Verification items for the finished model (mm, model axes). A direction names the side the tool comes from. Coordinates: 2 decimals unless noted, no trailing zeros. Order: outer loops, then holes, each group sorted by start corner. A loop starts at its lowest first (then second) coordinate and runs counter-clockwise, first axis right, second up. Notation, with made-up numbers: M 32.5,52 L 50.5,52 A30 ccw 50.5,80 Z; hole C 54.25,-25 d6. An arc over 180 degrees is marked long. Return JSON: item names as keys, results as strings. Group by question number.
Q1. Mould release check, pull along Y, two halves, no side actions. Record for faces 1 (the face through (8, -32.329, 4)), 2 (the face through (-36, 37.671, 4)), 3 (the face through (-36.58, 25.84, 2.46)): pulls with the +Y half, pulls with the -Y half, needs draft (parallel to the pull), parting line crosses it, or undercut.
Q2. Section check A-A, the plane x = -2.5. Enter the section's corners in (y, z), then the cut area to 4 significant figures.
Q3. Access from +Z, -Z, +X, -X, +Y, -Y to the whole of each face (thin tool, end or side, straight path). Record for faces 4 (the face through (30.98, 9.22, 4.42)), 5 (the face through (37.73, -28.88, 3.13)), 6 (the face through (14, -12, 2.5)).
Q4. Thickness scan on probe 1 along X at (y, z) = (7.75, 3.75); probe 2 along X at (y, z) = (-15, 4.5); probe 3 along Y at (x, z) = (-27.5, 3). Record the ranges inside material, lowest first.
Q5. Go/stop test with flat-tipped pins: pin 1 Ø4 at (x, z) = (67.61, 3.8) entering from +Y; pin 2 Ø19 at (x, y) = (-35.89, 17.67) entering from -Z; pin 3 Ø3 at (x, z) = (36.11, 3.8) entering from -Y; pin 4 Ø1.8 at (x, y) = (-35.89, 27.17) entering from +Z. Record where each tip stops, or that it passes through.
Q6. Section check B-B, the plane x = 48. Enter the section's corners in (y, z).
from build123d import *

# Parameters (mm, degrees)
BOSS_EXTRU_1_DEPTH       = 7.5
REPOSE_MOTEUR_DEPTH      = 8
ESQUISSE5_R              = 8
FIXATION_COURROI_1_DEPTH = 5
ESQUISSE6_R              = 5.5
FIXATION_COURROI_2_DEPTH = 2.5
ESQUISSE3_R              = 1.5
ESQUISSE3_R_2            = 6
FIXATION_MOTEUR_1_DEPTH  = 5
ESQUISSE2_R              = 13.5
FIXATION_MOTEUR_2_DEPTH  = 2.5
ESQUISSE9_R              = 1.75
PERCAGE_1_DEPTH          = 7
ESQUISSE7_R              = 1.75
PERCAGE_2_DEPTH          = 7


with BuildPart() as part:
    # Esquisse1 → Boss.-Extru.1 (new body)
    with BuildSketch(Plane.XY):
        Polygon((-53.385579659, 37.671052632), (-53.385579659, -32.328947368), (71.614420341, -32.328947368), (71.614420341, 12.671052632), (-18.385579659, 12.671052632), (-18.385579659, 37.671052632), align=None)
    extrude(amount=BOSS_EXTRU_1_DEPTH)

    # Esquisse4 → Repose moteur (cut)
    with BuildSketch(Plane.XY.offset(7.5)):
        with BuildLine():
            Line((41.534547933, 12.671052632), (66.614420341, 12.671052632))
            ThreePointArc((66.614420341, 12.671052632), (54.074484137, 4.171052632), (41.534547933, 12.671052632))
        make_face()
        with BuildLine():
            Line((-20.599533185, 7.678512609), (-33.878119681, -9.114993842))
            ThreePointArc((-33.878119681, -9.114993842), (-33.385579659, -13.328947368), (-29.171626132, -12.836407346))
            Line((-29.171626132, -12.836407346), (-15.893039636, 3.957099105))
            ThreePointArc((-15.893039636, 3.957099105), (-16.385579659, 8.171052632), (-20.599533185, 7.678512609))
        make_face()
    extrude(amount=-REPOSE_MOTEUR_DEPTH, mode=Mode.SUBTRACT)

    # Esquisse5 → Fixation courroi 1 (cut)
    with BuildSketch(Plane.XY.offset(7.5)):
        with Locations((8.614420341, -14.328947368)):
            Circle(ESQUISSE5_R)
    extrude(amount=-FIXATION_COURROI_1_DEPTH, mode=Mode.SUBTRACT)

    # Esquisse6 → Fixation courroi 2 (cut)
    with BuildSketch(Plane(origin=(0, 0, 0), x_dir=(-1, 0, 0), z_dir=(0, 0, -1))):
        with Locations((-8.614420341, -14.328947368)):
            Circle(ESQUISSE6_R)
    extrude(amount=-FIXATION_COURROI_2_DEPTH, mode=Mode.SUBTRACT)

    # Esquisse3 → Fixation moteur 1 (cut)
    with BuildSketch(Plane(origin=(0, 0, 0), x_dir=(-1, 0, 0), z_dir=(0, 0, -1))):
        with Locations((45.385579659, 17.671052632)):
            Circle(ESQUISSE3_R)
        with Locations((35.885579659, 8.171052632)):
            Circle(ESQUISSE3_R)
        with Locations((26.385579659, 17.671052632)):
            Circle(ESQUISSE3_R)
        with Locations((35.885579659, 27.171052632)):
            Circle(ESQUISSE3_R)
        with Locations((35.885579659, 17.671052632)):
            Circle(ESQUISSE3_R_2)
    extrude(amount=-FIXATION_MOTEUR_1_DEPTH, mode=Mode.SUBTRACT)

    # Esquisse2 → Fixation moteur 2 (cut)
    with BuildSketch(Plane.XY.offset(7.5)):
        with Locations((-35.885579659, 17.671052632)):
            Circle(ESQUISSE2_R)
    extrude(amount=-FIXATION_MOTEUR_2_DEPTH, mode=Mode.SUBTRACT)

    # Esquisse9 → Percage 1 (cut)
    with BuildSketch(Plane(origin=(0, 12.671052632, 0), x_dir=(1, 0, 0), z_dir=(0, 1, 0))):
        with Locations((-12.135579659, -3.75)):
            Circle(ESQUISSE9_R)
        with Locations((29.364420341, -3.75)):
            Circle(ESQUISSE9_R)
    extrude(amount=-PERCAGE_1_DEPTH, mode=Mode.SUBTRACT)

    # Esquisse7 → Percage 2 (cut)
    with BuildSketch(Plane.XZ.offset(32.328947368)):
        with Locations((-49.385579659, 3.800276617)):
            Circle(ESQUISSE7_R)
        with Locations((-17.885579659, 3.800276617)):
            Circle(ESQUISSE7_R)
        with Locations((36.114420341, 3.800276617)):
            Circle(ESQUISSE7_R)
        with Locations((67.614420341, 3.800276617)):
            Circle(ESQUISSE7_R)
    extrude(amount=-PERCAGE_2_DEPTH, mode=Mode.SUBTRACT)


solid = part.part
Numbers:
{
 "1": {"face 1": "pulls with the -Y half", "face 2": "pulls with the +Y half", "face 3": "undercut"},
 "2": {"outline": "M -32.33,0 L 12.67,0 L 12.67,7.5 L -32.33,7.5 Z", "area": "337.5 mm2"},
 "3": {"face 4": "+Y", "face 5": "-Y", "face 6": "+Z"},
 "4": {"probe 1": "x = -53.39 to -37.33, -34.45 to -20.54, -15.95 to -13.89, -10.39 to 27.61, 31.11 to 44.92, 63.23 to 71.61", "probe 2": "x = -53.39 to 0.64, 16.59 to 71.61", "probe 3": "y = -32.33 to -10.72, -1.05 to 16.67, 18.68 to 37.67"},
 "5": {"pin 1": "stops at y = 12.67", "pin 2": "stops at z = 0", "pin 3": "stops at y = -25.33", "pin 4": "passes through"},
 "6": {"outline": "M -32.33,0 L 5.61,0 L 5.61,7.5 L -32.33,7.5 Z"}
}
